Verification items for the finished model (mm, model axes). Face numbers are marked on the shaded views. A direction names the side the tool comes from. Round coordinates to 2 decimals unless told otherwise and drop trailing zeros. Write each loop counter-clockwise with the first axis right and the second up, starting at its lowest first coordinate (ties: lowest second). Pieces come first, ordered by that corner, then holes. Notation, with made-up numbers: M 13,-17.5 L 57,-17.5 A11 ccw 57,-11.5 Z; hole C 41.25,76.5 d7. An arc over 180 degrees is marked long. Use a Markdown table: item, result. Add a question column.
from build123d import *

# Parameters (mm, degrees)
F1_DEPTH = 5.9
F2_DEPTH = 16
F3_R     = 5.875
F3_R_2   = 4.85
F4_DEPTH = 2.5
F6_DEPTH = 20.5


with BuildPart() as f1:
    # F0 (on Front) → F1 (new body)
    with BuildSketch(Plane.XZ):
        with BuildLine():
            Line((-2.8142494559, -3.95), (2.8142494559, -3.95))
            ThreePointArc((2.8142494559, -3.95), (4.311125715, -2.2218674734), (4.85, 0))
            ThreePointArc((4.85, 0), (4.311125715, 2.2218674734), (2.8142494559, 3.95))
            Line((2.8142494559, 3.95), (-2.8142494559, 3.95))
            ThreePointArc((-2.8142494559, 3.95), (-4.85, 0), (-2.8142494559, -3.95))
        make_face()
        with BuildLine():
            ThreePointArc((-2.8142494559, -3.95), (0, -4.85), (2.8142494559, -3.95))
            Line((2.8142494559, -3.95), (-2.8142494559, -3.95))
        make_face()
        with BuildLine():
            Line((-2.8142494559, 3.95), (2.8142494559, 3.95))
            ThreePointArc((2.8142494559, 3.95), (0, 4.85), (-2.8142494559, 3.95))
        make_face()
    extrude(amount=-F1_DEPTH)

    # F0 (on Front) → F2 (join)
    with BuildSketch(Plane.XZ):
        with BuildLine():
            Line((-6.75, -3.95), (-2.8142494559, -3.95))
            ThreePointArc((-2.8142494559, -3.95), (-4.85, 0), (-2.8142494559, 3.95))
            Line((-2.8142494559, 3.95), (-6.75, 3.95))
            Line((-6.75, 3.95), (-6.75, -3.95))
        make_face()
        with BuildLine():
            Line((-2.8142494559, -3.95), (2.8142494559, -3.95))
            ThreePointArc((2.8142494559, -3.95), (4.311125715, -2.2218674734), (4.85, 0))
            ThreePointArc((4.85, 0), (4.311125715, 2.2218674734), (2.8142494559, 3.95))
            Line((2.8142494559, 3.95), (-2.8142494559, 3.95))
            ThreePointArc((-2.8142494559, 3.95), (-4.85, 0), (-2.8142494559, -3.95))
        make_face()
        with BuildLine():
            Line((2.8142494559, -3.95), (6.75, -3.95))
            Line((6.75, -3.95), (6.75, 3.95))
            Line((6.75, 3.95), (2.8142494559, 3.95))
            ThreePointArc((2.8142494559, 3.95), (4.311125715, 2.2218674734), (4.85, 0))
            ThreePointArc((4.85, 0), (4.311125715, -2.2218674734), (2.8142494559, -3.95))
        make_face()
    extrude(amount=F2_DEPTH)

    # F3 (on face) → F4 (join)
    with BuildSketch(Plane(origin=(0, 5.9, 0), x_dir=(-1, 0, 0), z_dir=(0, 1, 0))):
        Circle(F3_R)
        Circle(F3_R_2, mode=Mode.SUBTRACT)
        Circle(F3_R_2)
    extrude(amount=F4_DEPTH)

    # F5 (on face) → F6 (join)
    with BuildSketch(Plane(origin=(0, 8.4, 0), x_dir=(-1, 0, 0), z_dir=(0, 1, 0))):
        Polygon((-6.7360967927, -3.8890872965), (3.8890872965, -6.7360967927), (6.7360967927, 3.8890872965), (-3.8890872965, 6.7360967927), align=None)
    extrude(amount=F6_DEPTH)


solid = f1.part
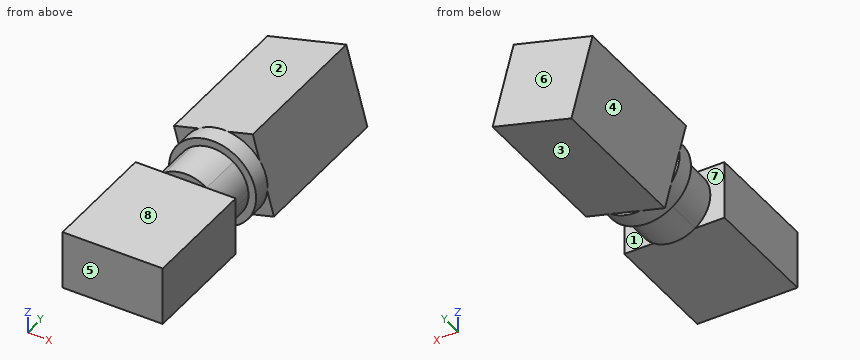
1. Access from +Z, -Z, +X, -X, +Y, -Y to the whole of each face (thin tool, end or side, straight path). Record for the marked faces 1, 2, 3 and 4.
2. Cross-section at A-A on x = -1.75. Enter the section's corners in (y, z).
3. Cross-section at B-B on y = 22. Enter the section's corners in (x, z), plus the area to 3 significant figures.
4. Depth check by flat-ended pin: pin 1 Ø4 at (x, y) = (-2, -11) entering from -Z; pin 2 Ø0.7 at (x, z) = (1, -4.5) entering from -Y; pin 3 Ø2.5 at (x, z) = (3.5, 5.5) entering from -Y. Enter the tip coordinate at first touch or a pass-through.
5. Release check for a two-part mould opening along Y. For the marked faces 5, 6, 7 and 8 record: +Y half, -Y half, draft (parallel to the pull), parting line (faces both ways), or undercut.
6. Scan lines: line 1 along Y through (x, z) = (5, -2); line 2 along Y through (x, z) = (-5.25, 3); line 3 along Y through (x, z) = (-3.5, -5.5). Record each from-to range of solid material in increasing order. Write a range as from..to.
7. Cross-section at D-D on y = -8. Enter the section's corners in (x, z), plus the area to 3 significant figures.
8. Cross-section at C-C on z = 2.75. Enter the section's corners in (x, y) (3 decimals).
Answer:
| question | item | result |
|---|---|---|
| 1 | face 1 | +X |
| 1 | face 2 | +Z, -X, +Y |
| 1 | face 3 | -Z, +X, +Y |
| 1 | face 4 | -Z, -X, +Y |
| 2 | outline | M -16,-3.95 L 0,-3.95 L 0,-4.52 L 5.9,-4.52 L 5.9,-5.61 L 8.4,-5.61 L 8.4,-6.16 L 28.9,-6.16 L 28.9,5.23 L 8.4,5.23 L 8.4,5.61 L 5.9,5.61 L 5.9,4.52 L 0,4.52 L 0,3.95 L -16,3.95 Z |
| 3 | outline | M -6.74,3.89 L -3.89,-6.74 L 6.74,-3.89 L 3.89,6.74 Z |
| 3 | area | 121 mm^2 |
| 4 | pin 1 | stops at z = -3.95 |
| 4 | pin 2 | stops at y = 0 |
| 4 | pin 3 | stops at y = 5.9 |
| 5 | face 5 | -Y half |
| 5 | face 6 | +Y half |
| 5 | face 7 | undercut |
| 5 | face 8 | draft |
| 6 | line 1 | y = -16..0, 5.9..28.9 |
| 6 | line 2 | y = -16..0, 8.4..28.9 |
| 6 | line 3 | y = 8.4..28.9 |
| 7 | outline | M -6.75,-3.95 L 6.75,-3.95 L 6.75,3.95 L -6.75,3.95 Z |
| 7 | area | 107 mm^2 |
| 8 | outline | M -6.75,-16 L 6.75,-16 L 6.75,0 L 3.995,0 L 3.995,5.9 L 5.192,5.9 L 5.192,8.4 L 4.957,8.4 L 4.957,28.9 L -6.431,28.9 L -6.431,8.4 L -5.192,8.4 L -5.192,5.9 L -3.995,5.9 L -3.995,0 L -6.75,0 Z |
